Autodesk Fusion 360 part; units mm, degrees
sketch "Sketch1" plane through (0, 0, 0) normal (0, 1, 0) x (1, 0, 0)
  line L0 (127, -22.25) -> (-127, -22.25)
  line L1 (-127, -22.25) -> (-127, 22.25)
  line L2 (-127, 22.25) -> (127, 22.25)
  line L3 (127, 22.25) -> (127, -22.25)
  line L4 (127, -22.25) -> (-127, 22.25) construction
  line L5 (-127, -22.25) -> (127, 22.25) construction
  line L6 (-127, -22.25) -> (-111.125, -22.25) construction
  line L7 (-111.125, -22.25) -> (-111.125, 22.25) construction
  line L8 (-111.125, 22.25) -> (-127, 22.25) construction
  line L9 (-127, 22.25) -> (-127, -22.25) construction
  line L10 (-127, -22.25) -> (-110, -22.25)
  line L11 (-110, -22.25) -> (-110, 22.25)
  line L12 (-110, 22.25) -> (-127, 22.25)
  line L13 (-127, 22.25) -> (-127, -22.25)
  line L14 (-127, -22.25) -> (-111.125, 22.25) construction
  circle A0 centre (-119.0625, 0) radius 2.6
  circle A1 centre (-119.0625, 0) radius 2.5 construction
  circle A2 centre (-119.0625, -15.875) radius 2.6
  circle A3 centre (-119.0625, 15.875) radius 2.6
  line L15 (0, -22.25) -> (0, 22.25) construction
  circle A4 centre (119.0625, -15.875) radius 2.6
  line L16 (127, 22.25) -> (127, -22.25)
  line L17 (111.125, -22.25) -> (111.125, 22.25) construction
  line L18 (127, -22.25) -> (111.125, 22.25) construction
  line L19 (127, -22.25) -> (127, 22.25)
  line L20 (110, -22.25) -> (110, 22.25)
  line L21 (127, -22.25) -> (111.125, -22.25) construction
  circle A5 centre (119.0625, 0) radius 2.5 construction
  line L22 (111.125, 22.25) -> (127, 22.25) construction
  circle A6 centre (119.0625, 15.875) radius 2.6
  line L23 (110, 22.25) -> (127, 22.25)
  line L24 (127, 22.25) -> (127, -22.25) construction
  circle A7 centre (119.0625, 0) radius 2.6
  line L25 (127, -22.25) -> (110, -22.25)
  dimension "d1" = 254
  dimension "d2" = 44.5
  dimension "d3" = 15.875
  dimension "d4" = 17
  dimension "d5" = 5.2
  dimension "d9" = 0
  dimension "d10" = 15.875
  dimension "d18" = 15.875
extrude "Extrude1" add sketch "Sketch1" along normal blind 4
extrude "Extrude2" add sketch "Sketch1" along normal blind 6 contours L0 L2 L11 L20
fillet "Fillet1" radius 4 4 edges at (127, 2, 22.25) (127, 2, -22.25) (-127, 2, -22.25) (-127, 2, 22.25)
sketch "Sketch2" plane through (0, 0, 0) normal (0, 1, 0) x (1, 0, 0)
  line L0 (0, 13) -> (-42.5625, 13)
  line L1 (-42.5625, 13) -> (-42.5625, 18.0675)
  line L2 (-42.5625, 18.0675) -> (0, 18.0675)
  line L3 (0, 18.0675) -> (0, 13)
  line L4 (0, 13) -> (42.5073, 13)
  line L5 (42.5073, 13) -> (42.5073, 18.0969)
  line L6 (42.5073, 18.0969) -> (0, 18.0969)
  line L7 (0, 18.0969) -> (0, 13)
extrude "Extrude3" cut sketch "Sketch2" along normal blind 460
extrude "Extrude4" cut 1 faces at (-28.375, 4, -18.0675) along direction (0, 0, -1) blind 0.03
sketch "Sketch3" plane through (0, 6, 0) normal (0, 1, 0) x (-1, 0, 0)
  line L0 (0, -18.0975) -> (0, -18.0969)
  line L1 (0, -18.0969) -> (-42.5073, -18.0969)
  line L2 (-42.5073, -18.0969) -> (-42.5073, -13)
  line L3 (-42.5073, -13) -> (42.5625, -13)
  line L4 (42.5625, -13) -> (42.5625, -18.0975)
  line L5 (42.5625, -18.0975) -> (0, -18.0975)
  line L6 (110, 22.25) -> (-110, 22.25)
  line L7 (-110, 22.25) -> (-110, -22.25)
  line L8 (-110, -22.25) -> (110, -22.25)
  line L9 (110, -22.25) -> (110, 22.25)
  line L10 (-45, -10) -> (45, -10)
  line L11 (45, -10) -> (45, -20)
  line L12 (45, -20) -> (-45, -20)
  line L13 (-45, -20) -> (-45, -10)
extrude "Extrude5" add sketch "Sketch3" along normal blind 12 contours L10 L11 L12 L13
sketch "Sketch4" plane through (0, 0, 0) normal (0, -1, 0) x (1, 0, 0)
  arc A0 (-123, 22.25) -> (-127, 18.25) centre (-123, 18.25) ccw
  line L0 (-127, 18.25) -> (-127, -18.25)
  arc A1 (-127, -18.25) -> (-123, -22.25) centre (-123, -18.25) ccw
  line L1 (-123, -22.25) -> (123, -22.25)
  arc A2 (123, -22.25) -> (127, -18.25) centre (123, -18.25) ccw
  line L2 (127, -18.25) -> (127, 18.25)
  arc A3 (127, 18.25) -> (123, 22.25) centre (123, 18.25) ccw
  line L3 (123, 22.25) -> (-123, 22.25)
  circle A4 centre (119.0625, 0) radius 2.6
  circle A5 centre (119.0625, 15.875) radius 2.6
  circle A6 centre (119.0625, -15.875) radius 2.6
  circle A7 centre (-119.0625, 15.875) radius 2.6
  circle A8 centre (-119.0625, -15.875) radius 2.6
  circle A9 centre (-119.0625, 0) radius 2.6
  line L4 (0, -18.0969) -> (0, -18.0975)
  line L5 (0, -18.0975) -> (-42.5625, -18.0975)
  line L6 (-42.5625, -18.0975) -> (-42.5625, -13)
  line L7 (-42.5625, -13) -> (42.5073, -13)
  line L8 (42.5073, -13) -> (42.5073, -18.0969)
  line L9 (42.5073, -18.0969) -> (0, -18.0969)
  circle A10 centre (0, 21) radius 1.4142
  line L10 (-1.4142, 21.0088) -> (-1.4065, 22.25)
  line L11 (1.4142, 21.0088) -> (1.4065, 22.25)
extrude "Extrude6" cut sketch "Sketch4" against normal blind 11.5 contours L3 A10 L10 | L3 A10 | L3 A10 L11 picked at (-0.1575, 22.3211)
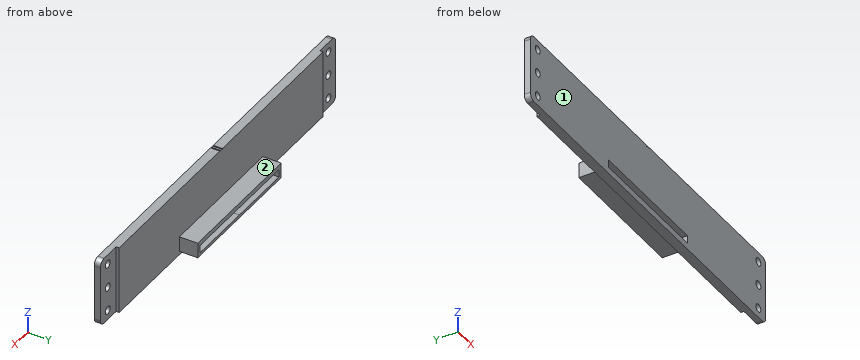
The model under review builds one solid part; all positions refer to its coordinate system, in mm. Face numbers are marked on the shaded views. A direction names the side the tool comes from. Round coordinates to 2 decimals unless told otherwise and drop trailing zeros. Loops run counter-clockwise (first coordinate to the right, second up) from the corner with the lowest first, then second, coordinate; pieces in that order, holes last. Notation, with made-up numbers: (83, 45) -> (104, 45) arc R17 ccw to (104, 65) -> close; hole circle Ø8 at (-39.5, 59.5). An arc over 180 degrees is marked (long way). Write item = value, one per line. Start each with the question number.
Item 1: Take a section at C-C on x = 77. Give the boundary of the cut face in (y, z).
Item 2: For the marked faces 1 and 2, list the 3-axis set-ups (+Z, -Z, +X, -X, +Y, -Y) from which the entire face can be reached by the end or side of a thin tool; tool diameter is ignored.
Item 3: Take a section at A-A on y = 15.5. Give the boundary of the cut face in (x, z).
Item 4: Take a section at D-D on z = 11. Give the boundary of the cut face in (x, y), plus the area to 3 significant figures.
Item 5: To check wall thickness, follow L1, parallel to X at y = 2.25, z = 0; L2, parallel to Z at x = -15, y = 4; L3, parallel to Z at x = 20.5, y = 6.25. State the ranges of each line that lie inside material, in increasing order.
Item 6: Insertion check: pin 1 (7 mm diameter, centred on x = -119.06, z = 0, fed in from -Y); pin 2 (1.6 mm diameter, centred on y = 5.5, z = 9, fed in from +X); pin 3 (3 mm diameter, centred on y = 14, z = -13.5, fed in from -X); pin 4 (18.5 mm diameter, centred on x = -116, z = 9, fed in from +Y). Each pin has a flat end and moves straight along its axis. Give the tip position at first contact, or say it passes through.
Item 7: Take a section at B-B on z = 0. Give the boundary of the cut face in (x, y).
Result:
q1.outline = (0, -22.25) -> (6, -22.25) -> (6, 22.25) -> (0, 22.25) -> close
q2.face_1 = +Z, -Z, +X, -X, -Y
q2.face_2 = +Z, +X, -X, +Y
q3.outline = (-45, -20) -> (45, -20) -> (45, -10) -> (-45, -10) -> close; hole (-42.56, -18.1) -> (0, -18.1) -> (42.51, -18.1) -> (42.51, -13) -> (-42.56, -13) -> close
q4.outline = (-127, 0) -> (127, 0) -> (127, 4) -> (110, 4) -> (110, 6) -> (-110, 6) -> (-110, 4) -> (-127, 4) -> close
q4.area = 1,460 mm²
q5.L1 = -127 to -121.66, -116.46 to 116.46, 121.66 to 127
q5.L2 = -22.25 to -18.1, -13 to 22.25
q5.L3 = -20 to -18.1, -13 to -10
q6.pin_1 = 0
q6.pin_2 = 110
q6.pin_3 = -45
q6.pin_4 = 6
q7.outline = (-127, 0) -> (-121.66, 0) -> (-121.66, 4) -> (-127, 4) -> close; (-116.46, 0) -> (116.46, 0) -> (116.46, 4) -> (110, 4) -> (110, 6) -> (-110, 6) -> (-110, 4) -> (-116.46, 4) -> close; (121.66, 0) -> (127, 0) -> (127, 4) -> (121.66, 4) -> close
